Source: CAD feature listing. Evaluate the final solid. Frame: model axes, mm. A direction names the side the tool comes from. Give positions to 0.01 mm unless a question says otherwise; leave off trailing zeros. Write each loop counter-clockwise with the first axis right and the second up, starting at its lowest first coordinate (ties: lowest second). Pieces come first, ordered by that corner, then holes.
```python
from build123d import *

# Parameters (mm, degrees)
SKETCH1_W                       = 39
SKETCH1_H                       = 40
BOSS_EXTRUDE1_DEPTH             = 10
SM1_THREADED_HOLE_REACH         = 12
SKETCH1_3_R                     = 12.8397
OVERSIZED_8_32_THRU_HOLES_REACH = 12
SKETCH1_4_R                     = 3.35
F_8_32_TAPPED_HOLE1_D           = 3.4544
F_8_32_TAPPED_HOLE1_DEPTH       = 6
F_8_32_TAPPED_HOLE1_TIP         = 1.037806461


with BuildPart() as part:
    # Sketch1 → Boss-Extrude1 (new body)
    with BuildSketch(Plane(origin=(0, 0, 0), x_dir=(0, 0, -1), z_dir=(1, 0, 0))):
        with Locations((3.409258695, -8.993814604)):
            Rectangle(SKETCH1_W, SKETCH1_H)
    extrude(amount=BOSS_EXTRUDE1_DEPTH)

    # Sketch1_3 → SM1 threaded hole (cut, up to next)
    with BuildSketch(Plane(origin=(0, 0, 0), x_dir=(0, 0, -1), z_dir=(1, 0, 0)), mode=Mode.PRIVATE) as sm1_threaded_hole_sk1:
        with Locations((3.409258695, -8.993814604)):
            Circle(SKETCH1_3_R)
    sm1_threaded_hole_tool1 = extrude(sm1_threaded_hole_sk1.sketch, amount=SM1_THREADED_HOLE_REACH, mode=Mode.PRIVATE) & part.part
    add(sm1_threaded_hole_tool1.solids().sort_by_distance((0, -8.993815, -3.409259))[0], mode=Mode.SUBTRACT)

    # Sketch1_4 → oversized 8-32 thru holes (cut, up to next)
    with BuildSketch(Plane(origin=(0, 0, 0), x_dir=(0, 0, -1), z_dir=(1, 0, 0)), mode=Mode.PRIVATE) as oversized_8_32_thru_holes_sk1:
        with Locations((-10.590741305, 5.006185396)):
            Circle(SKETCH1_4_R)
    oversized_8_32_thru_holes_tool1 = extrude(oversized_8_32_thru_holes_sk1.sketch, amount=OVERSIZED_8_32_THRU_HOLES_REACH, mode=Mode.PRIVATE) & part.part
    add(oversized_8_32_thru_holes_tool1.solids().sort_by_distance((0, 5.006185, 10.590741))[0], mode=Mode.SUBTRACT)
    # Sketch1_4 → oversized 8-32 thru holes (cut, up to next)
    with BuildSketch(Plane(origin=(0, 0, 0), x_dir=(0, 0, -1), z_dir=(1, 0, 0)), mode=Mode.PRIVATE) as oversized_8_32_thru_holes_sk2:
        with Locations((17.409258695, 5.006185396)):
            Circle(SKETCH1_4_R)
    oversized_8_32_thru_holes_tool2 = extrude(oversized_8_32_thru_holes_sk2.sketch, amount=OVERSIZED_8_32_THRU_HOLES_REACH, mode=Mode.PRIVATE) & part.part
    add(oversized_8_32_thru_holes_tool2.solids().sort_by_distance((0, 5.006185, -17.409259))[0], mode=Mode.SUBTRACT)
    # Sketch1_4 → oversized 8-32 thru holes (cut, up to next)
    with BuildSketch(Plane(origin=(0, 0, 0), x_dir=(0, 0, -1), z_dir=(1, 0, 0)), mode=Mode.PRIVATE) as oversized_8_32_thru_holes_sk3:
        with Locations((17.409258695, -22.993814604)):
            Circle(SKETCH1_4_R)
    oversized_8_32_thru_holes_tool3 = extrude(oversized_8_32_thru_holes_sk3.sketch, amount=OVERSIZED_8_32_THRU_HOLES_REACH, mode=Mode.PRIVATE) & part.part
    add(oversized_8_32_thru_holes_tool3.solids().sort_by_distance((0, -22.993815, -17.409259))[0], mode=Mode.SUBTRACT)
    # Sketch1_4 → oversized 8-32 thru holes (cut, up to next)
    with BuildSketch(Plane(origin=(0, 0, 0), x_dir=(0, 0, -1), z_dir=(1, 0, 0)), mode=Mode.PRIVATE) as oversized_8_32_thru_holes_sk4:
        with Locations((-10.590741305, -22.993814604)):
            Circle(SKETCH1_4_R)
    oversized_8_32_thru_holes_tool4 = extrude(oversized_8_32_thru_holes_sk4.sketch, amount=OVERSIZED_8_32_THRU_HOLES_REACH, mode=Mode.PRIVATE) & part.part
    add(oversized_8_32_thru_holes_tool4.solids().sort_by_distance((0, -22.993815, 10.590741))[0], mode=Mode.SUBTRACT)

    # 8-32 Tapped Hole1
    with Locations(Plane(origin=(0, -28.993814604, 0), x_dir=(-1, 0, 0), z_dir=(0, -1, 0))):
        with Locations((-5, 9.909258695)):
            Hole(F_8_32_TAPPED_HOLE1_D / 2, depth=F_8_32_TAPPED_HOLE1_DEPTH)
            with Locations((0, 0, -(F_8_32_TAPPED_HOLE1_DEPTH + F_8_32_TAPPED_HOLE1_TIP / 2))):  # 118° drill point
                Cone(0, F_8_32_TAPPED_HOLE1_D / 2, F_8_32_TAPPED_HOLE1_TIP, mode=Mode.SUBTRACT)


solid = part.part
```
1. Cut plane A-A, the plane z = -5.5. Return the cut outline in (x, y).
2. Access query for faces 1 (the cylindrical face through (4.93, -22.847, 13.938)), 2 (the cylindrical face through (3.6, -26, -8.9)). Directions: +Z, -Z, +X, -X, +Y, -Y. A direction counts if a zero-diameter tool reaches every point of the face in a straight line with its end or side. Return the directions, or none.
3. Cut plane D-D, the plane y = 0. Return the cut outline in (x, z), then the cut area to 3 significant figures.
4. Line query: L1, parallel to Z at x = 9.75, y = -23; L2, parallel to Y at x = 8.25, z = 10.5; L3, parallel to Y at x = 4.5, z = 7.5. Output: solid intervals per line, ascending.
5. Contact query for a flat-ended pin moving along its axis: P1, Ø6, axis at y = -22.99, z = 10.59, coming from the -X side (3 decimals). Output: stop coordinate, or through.
6. Mould query, pull axis Y, two halves, no side actions, for faces 3 (the flat face through (5, 11.006, -3)), 4 (the cylindrical face through (4.93, -21.53, -0.63)), 5 (the flat face through (5, -28.994, -3)), 6 (the flat face through (5, -9, 16.091)). Classes: +Y half, -Y half, draft (parallel to the pull), parting line (faces both ways), or undercut.
7. Cut plane C-C, the plane z = 12. Return the cut outline in (x, y).
8. Cut plane B-B, the plane y = -24.5. Return the cut outline in (x, z), then the cut area to 3 significant figures.
Response values:
1. outline: (0, -28.99) - (10, -28.99) - (10, -21.66) - (0, -21.66) - close; (0, 3.67) - (10, 3.67) - (10, 11.01) - (0, 11.01) - close
2. face 1: +X, -X
2. face 2: -Y
3. outline: (0, -22.91) - (10, -22.91) - (10, -12.57) - (0, -12.57) - close; (0, 5.75) - (10, 5.75) - (10, 16.09) - (0, 16.09) - close
3. area: 207 mm2
4. L1: z = -22.91 to -20.76, -14.06 to 7.24, 13.94 to 16.09
4. L2: y = -28.99 to -26.34, -19.65 to 1.66, 8.35 to 11.01
4. L3: y = -28.99 to -24.29, -21.7 to -15.76, -2.22 to 3.71, 6.3 to 11.01
5. P1: passes through
6. face 3: +Y half
6. face 4: undercut
6. face 5: -Y half
6. face 6: draft
7. outline: (0, -28.99) - (10, -28.99) - (10, -26.03) - (0, -26.03) - close; (0, -19.95) - (10, -19.95) - (10, 1.97) - (0, 1.97) - close; (0, 8.05) - (10, 8.05) - (10, 11.01) - (0, 11.01) - close
8. outline: (0, -22.91) - (10, -22.91) - (10, -20.4) - (0, -20.4) - close; (0, -14.42) - (10, -14.42) - (10, 7.6) - (0, 7.6) - close; (0, 13.58) - (10, 13.58) - (10, 16.09) - (0, 16.09) - close; hole circle Ø3.45 at (5, -9.91)
8. area: 261 mm2
